The drawing under review shows one solid part. Ordinate dimensions are in mm from its lowest x, y, z. Coordinates: 2 decimals unless noted, no trailing zeros. Order: outer loops, then holes, each group sorted by start corner. A loop starts at its lowest first (then second) coordinate and runs counter-clockwise, first axis right, second up. Notation, with made-up numbers: (-18.75, 41) -> (24.25, 41) arc R26 cw to (24.25, 62) -> close; hole circle Ø3 at (-8, -36). An arc over 180 degrees is marked (long way). Use a Markdown table: item, result. Add a question column.
Q1. Wall thickness on probe 1 along X at (y, z) = (0.65, 65); probe 2 along X at (y, z) = (0.85, 33); probe 3 along Z at (x, y) = (8, 1.25): over which ranges is each line inside the solid? List them lowest first.
Q2. Add section A-A (z = 38.1). Count the separate pieces of the cut face and the enclosed holes in it, then the cut area to 3 significant figures.
Q3. Add section C-C (x = 10.5). State the section outline as (y, z) points (3 decimals).
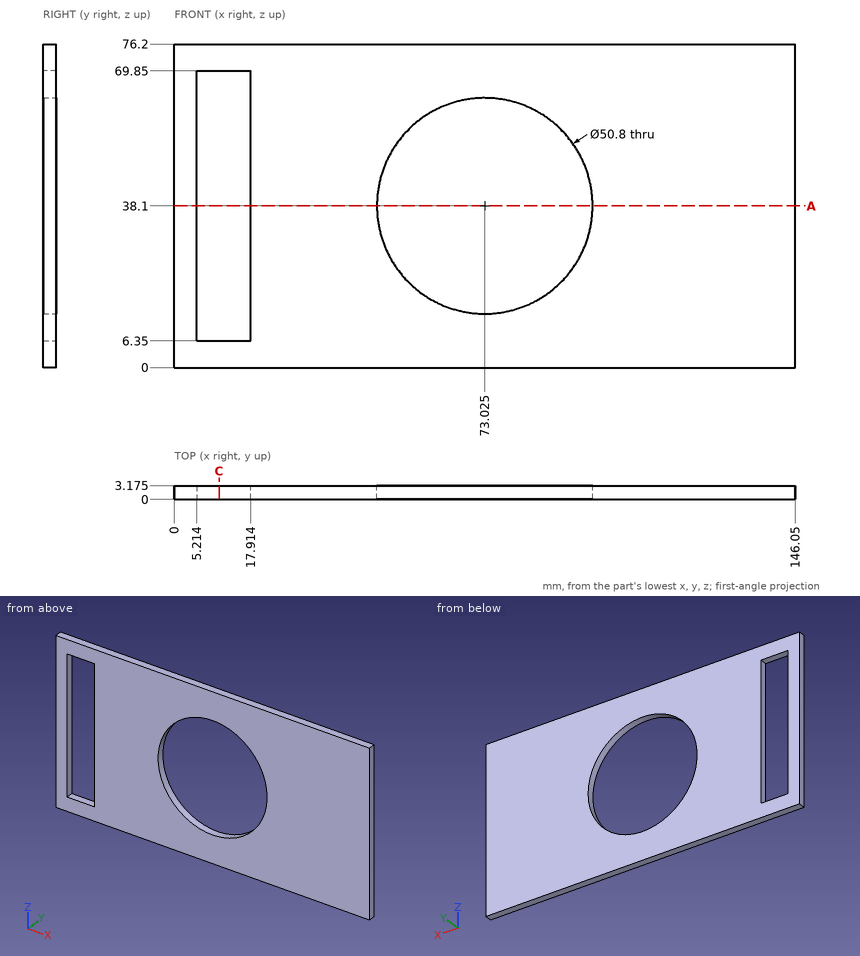
Established:
| question | item | result |
|---|---|---|
| 1 | probe 1 | 0 to 5.21, 17.91 to 146.05 |
| 1 | probe 2 | 0 to 5.21, 17.91 to 48.14, 97.91 to 146.05 |
| 1 | probe 3 | 0 to 6.35, 69.85 to 76.2 |
| 2 | separate pieces | 3 |
| 2 | enclosed holes | 0 |
| 2 | area | 262 mm^2 |
| 3 | outline | (0, 0) -> (3.175, 0) -> (3.175, 6.35) -> (0, 6.35) -> close; (0, 69.85) -> (3.175, 69.85) -> (3.175, 76.2) -> (0, 76.2) -> close |
